Design review of the part shown in the three views and the two pictorial views. Dimensions are in mm from the part's minimum x, y and z. Give positions to 0.01 mm unless a question says otherwise; leave off trailing zeros. Order: outer loops, then holes, each group sorted by start corner. A loop starts at its lowest first (then second) coordinate and runs counter-clockwise, first axis right, second up. Notation, with made-up numbers: (50.5, 82.5) - (81.5, 82.5) arc R23 ccw to (81.5, 111.5) - close; hole circle Ø4 at (82.25, 63). An arc over 180 degrees is marked (long way). Put each result on its own line as item: value.
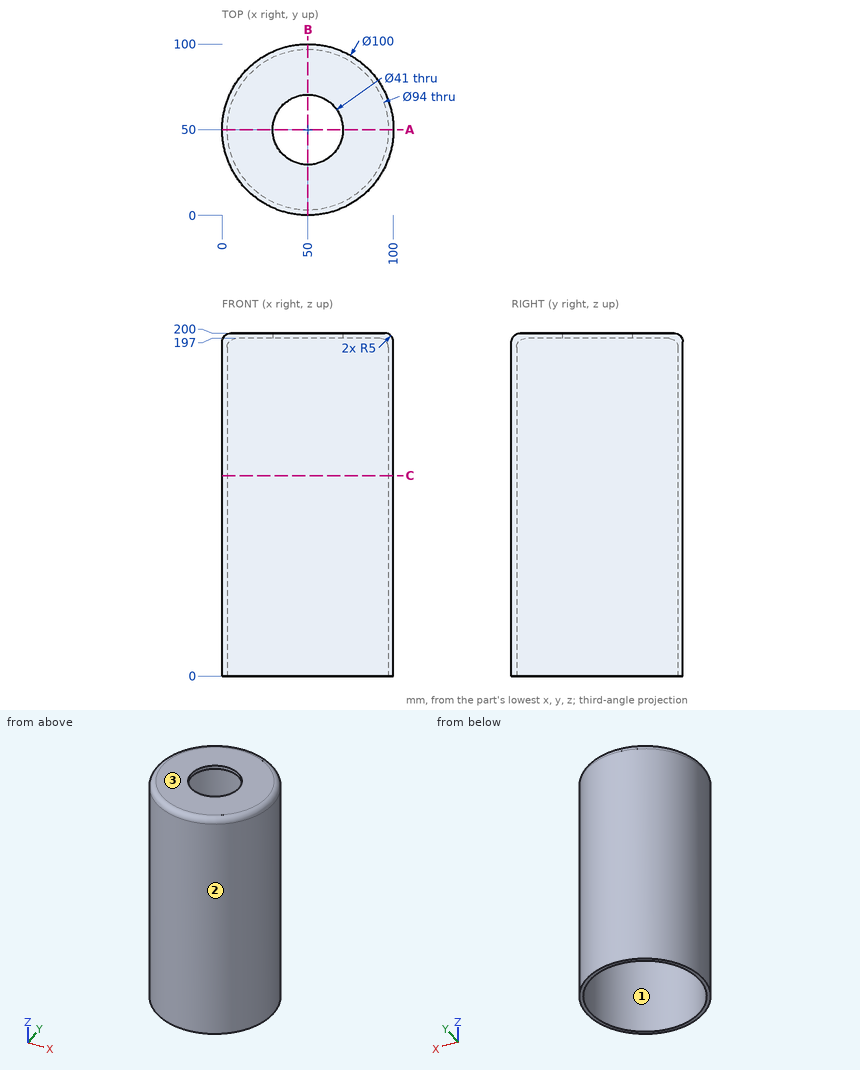
(1) Take a section at A-A, the plane y = 50. Write out the cut boundary in (x, z), then the cut area to 3 significant figures.
The answers:
outline: (0, 0) - (3, 0) - (3, 192) arc R5 cw to (8, 197) - (29.5, 197) - (29.5, 200) - (5, 200) arc R5 ccw to (0, 195) - close; (70.5, 197) - (92, 197) arc R5 cw to (97, 192) - (97, 0) - (100, 0) - (100, 195) arc R5 ccw to (95, 200) - (70.5, 200) - close
area: 1,360 mm^2
(2) Take a section at C-C, the plane z = 117. Write out the cut boundary in (x, y).
The answers:
outline: circle Ø100 at (50, 50); hole circle Ø94 at (50, 50)
(3) The part is to be moulded in two halves that separate along X. For the marked faces 1, 2 and 3, say which applies: pulls with the +X half, pulls with the -X half, needs draft (parallel to the pull), parting line crosses it, or undercut.
The answers:
face 1: undercut
face 2: parting line crosses it
face 3: needs draft
(4) Clearance check with flat-ended pins moving along their axes: pin 1 Ø3 at (x, y) = (17, 36.5) entering from -Z; pin 2 Ø3 at (x, z) = (57.5, 34) entering from -Y; pin 3 Ø12 at (y, z) = (77.5, 127) entering from -X. State where each tip first meets the part, or that it passes through.
The answers:
pin 1: z = 197
pin 2: y = 0.36
pin 3: x = 4.86
(5) Wall thickness on L1, parallel to Y at x = 52, z = 82; L2, parallel to X at y = 50, z = 74.5; L3, parallel to Z at x = 25, y = 62.5: over which ranges is each line inside the solid? List them lowest first.
The answers:
L1: 0.04 to 3.04, 96.96 to 99.96
L2: 0 to 3, 97 to 100
L3: 197 to 200
